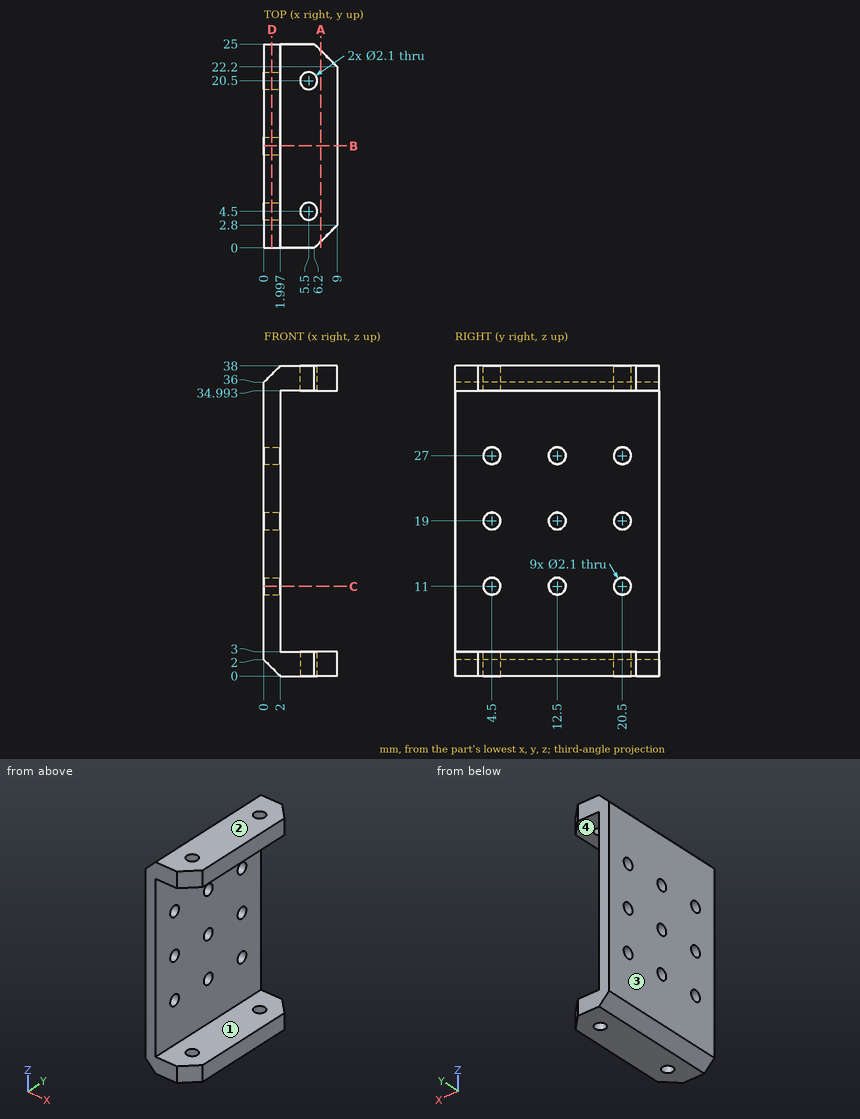
The drawing under review shows one solid part. Ordinate dimensions are in mm from its lowest x, y, z. Round coordinates to 2 decimals unless told otherwise and drop trailing zeros. Write each loop counter-clockwise with the first axis right and the second up, starting at its lowest first coordinate (ties: lowest second). Pieces come first, ordered by that corner, then holes. Notation, with made-up numbers: (55.25, 75.5) -> (89.25, 75.5) arc R27 cw to (89.25, 95.5) -> close; hole circle Ø6 at (89.5, -9). An arc over 180 degrees is marked (long way). One line per question, with ' | ' between items. Start each with the question number.
(1) Add section C-C, the plane z = 11. Write out the cut boundary in (x, y).
(2) Insertion check: P1, Ø2, axis at x = 7.5, z = 5.5, coming from the +Y side; P2, Ø5, axis at y = 9, z = 31.5, coming from the +X side. Each pin has a flat end and moves straight along its axis. Give the tip position at first contact, or say it passes through.
(3) Mouldability with a two-part tool opening along Z and no side actions: class the marked faces 1, 2, 3 and 4 as released by +Z, released by -Z, zero draft, split by the parting line, or undercut.
(4) Add section D-D, the plane x = 1. Give the number of separate pieces and of enclosed holes in the cut face, plus the area to 3 significant figures.
(5) For line 1 along Y through (x, z) = (5.5, 36.2); line 2 along Y through (x, z) = (0.8, 27); line 3 along Z through (x, y) = (2.75, 9.5), list the stretches that pass through material, from the lowest coordinate up. Write a range as from..to.
(6) Add section A-A, the plane x = 7. Write out the cut boundary in (y, z).
(7) Add section B-B, the plane y = 12.5. Write out the cut boundary in (x, z).
Answer list:
1) outline: (0, 0) -> (2, 0) -> (2, 3.45) -> (0, 3.45) -> close; (0, 5.55) -> (2, 5.55) -> (2, 11.45) -> (0, 11.45) -> close; (0, 13.55) -> (2, 13.55) -> (2, 19.45) -> (0, 19.45) -> close; (0, 21.55) -> (2, 21.55) -> (2, 25) -> (0, 25) -> close
2) P1: through | P2: x = 2
3) face 1: undercut | face 2: released by +Z | face 3: zero draft | face 4: undercut
4) separate pieces: 1 | enclosed holes: 9 | area: 869 mm²
5) line 1: 0..3.45, 5.55..19.45, 21.55..25 | line 2: 0..3.45, 5.55..11.45, 13.55..19.45, 21.55..25 | line 3: 0..3, 34.99..38
6) outline: (0.8, 0) -> (24.2, 0) -> (24.2, 3) -> (0.8, 3) -> close; (0.8, 34.99) -> (24.2, 34.99) -> (24.2, 38) -> (0.8, 38) -> close
7) outline: (0, 2) -> (2, 0) -> (9, 0) -> (9, 3) -> (2, 3) -> (2, 9.95) -> (0, 9.95) -> close; (0, 12.05) -> (2, 12.05) -> (2, 17.95) -> (0, 17.95) -> close; (0, 20.05) -> (2, 20.05) -> (2, 25.95) -> (0, 25.95) -> close; (0, 28.05) -> (2, 28.05) -> (2, 34.99) -> (9, 34.99) -> (9, 38) -> (2, 38) -> (0, 36) -> close
